```python
from build123d import *

# Parameters (mm, degrees)
ESBO_O1_R                = 87
RESSALTO_EXTRUS_O1_DEPTH = 2.5
CORTE_EXTRUS_O1_DEPTH    = 2.5
CORTE_EXTRUS_O2_START    = -2.5
ESBO_O3_W                = 27.5
ESBO_O3_H                = 33
CORTE_EXTRUS_O2_DEPTH    = 2.5
FILETE2_R                = 2
ESBO_O4_R                = 17
CORTE_EXTRUS_O3_DEPTH    = 4
CORTE_EXTRUS_O5_DEPTH    = 3
FURO_ROSCADO_DE_M2_51_D  = 2.05


with BuildPart() as part:
    # Esboço1 → Ressalto-extrusão1 (new body)
    with BuildSketch(Plane(origin=(0, 0, 0), x_dir=(1, 0, 0), z_dir=(0, 1, 0))):
        with Locations(Location((0, 0, 0), (0, 0, 270))):
            Circle(ESBO_O1_R)
    extrude(amount=RESSALTO_EXTRUS_O1_DEPTH)

    # Esboço2 → Corte-extrusão1 (cut)
    with BuildSketch(Plane(origin=(0, 2.5, 0), x_dir=(1, 0, 0), z_dir=(0, 1, 0))):
        Polygon((66.645866551, 55.922522043), (82.394162989, 37.154433186), (79.696950599, 34.891203265), (72.036506168, 28.463327168), (40.539913293, 65.999504881), (48.200357724, 72.427380978), (50.897570114, 74.690610899), align=None)
        Polygon((50.897570114, -74.690610899), (82.394162989, -37.154433186), (79.696950599, -34.891203265), (72.036506168, -28.463327168), (40.539913293, -65.999504881), (48.200357724, -72.427380978), align=None)
        Polygon((-72.036506168, 28.463327168), (-40.539913293, 65.999504881), (-48.200357724, 72.427380978), (-50.897570114, 74.690610899), (-66.645866551, 55.922522043), (-82.394162989, 37.154433186), (-79.696950599, 34.891203265), align=None)
        Polygon((-79.696950599, -34.891203265), (-82.394162989, -37.154433186), (-50.897570114, -74.690610899), (-48.200357724, -72.427380978), (-40.539913293, -65.999504881), (-72.036506168, -28.463327168), align=None)
    extrude(amount=-CORTE_EXTRUS_O1_DEPTH, mode=Mode.SUBTRACT)

    # Esboço3 → Corte-extrusão2 (cut)
    with BuildSketch(Plane(origin=(0, 2.5, 0), x_dir=(1, 0, 0), z_dir=(0, 1, 0)).offset(CORTE_EXTRUS_O2_START)):
        with Locations((-13.75, 58.5)):
            Rectangle(ESBO_O3_W, ESBO_O3_H)
        with Locations((13.75, 58.5)):
            Rectangle(ESBO_O3_W, ESBO_O3_H)
        with BuildLine():
            Line((0, 87), (0, 75))
            Line((0, 75), (27.5, 75))
            Line((27.5, 75), (44.09081537, 75))
            ThreePointArc((44.09081537, 75), (22.847319318, 83.946411478), (0, 87))
        make_face()
        with BuildLine():
            Line((-27.5, 75), (0, 75))
            Line((0, 75), (0, 87))
            ThreePointArc((0, 87), (-22.847319318, 83.946411478), (-44.09081537, 75))
            Line((-44.09081537, 75), (-27.5, 75))
        make_face()
    extrude(amount=CORTE_EXTRUS_O2_DEPTH, mode=Mode.SUBTRACT)

    # Filete2
    filete2_edges = [part.edges().sort_by_distance(p)[0] for p in [
        (27.5, 1.25, -42),
        (-27.5, 1.25, -42),
        (-27.5, 1.25, -75),
        (-44.09081537, 1.25, -75),
        (44.09081537, 1.25, -75),
        (27.5, 1.25, -75),
        (79.696950599, 1.25, 34.891203265),
        (72.036506168, 1.25, 28.463327168),
        (48.200357724, 1.25, 72.427380978),
        (40.539913293, 1.25, 65.999504881),
        (-79.696950599, 1.25, -34.891203265),
        (-72.036506168, 1.25, -28.463327168),
        (-48.200357724, 1.25, -72.427380978),
        (-40.539913293, 1.25, -65.999504881),
        (-79.696950599, 1.25, 34.891203265),
        (-48.200357724, 1.25, 72.427380978),
        (-40.539913293, 1.25, 65.999504881),
        (-72.036506168, 1.25, 28.463327168),
        (79.696950599, 1.25, -34.891203265),
        (48.200357724, 1.25, -72.427380978),
        (40.539913293, 1.25, -65.999504881),
        (72.036506168, 1.25, -28.463327168),
    ]]
    fillet(filete2_edges, radius=FILETE2_R)

    # Esboço4 → Corte-extrusão3 (cut)
    with BuildSketch(Plane(origin=(0, 2.5, 0), x_dir=(1, 0, 0), z_dir=(0, 1, 0))):
        with Locations(Location((61, 0, 0), (0, 0, 270))):
            Circle(ESBO_O4_R)
        with Locations(Location((-61, 0, 0), (0, 0, 270))):
            Circle(ESBO_O4_R)
    extrude(amount=-CORTE_EXTRUS_O3_DEPTH, mode=Mode.SUBTRACT)

    # Esboço7 → Corte-extrusão5 (cut)
    with BuildSketch(Plane(origin=(0, 2.5, 0), x_dir=(1, 0, 0), z_dir=(0, 1, 0))):
        with BuildLine():
            Line((-40.056146338, -19.904321081), (-26.557606535, -35.991254386))
            ThreePointArc((-26.557606535, -35.991254386), (-25.199829134, -36.698068563), (-23.739942429, -36.237768053))
            Line((-23.739942429, -36.237768053), (-7.653009124, -22.73922825))
            ThreePointArc((-7.653009124, -22.73922825), (-6.946194947, -21.381450849), (-7.406495457, -19.921564144))
            Line((-7.406495457, -19.921564144), (-20.90503526, -3.834630839))
            ThreePointArc((-20.90503526, -3.834630839), (-22.262812661, -3.127816662), (-23.722699366, -3.588117172))
            Line((-23.722699366, -3.588117172), (-39.809632672, -17.086656975))
            ThreePointArc((-39.809632672, -17.086656975), (-40.516446848, -18.444434376), (-40.056146338, -19.904321081))
        make_face()
        with BuildLine():
            Line((-23.722699366, 3.588117172), (-39.809632672, 17.086656975))
            ThreePointArc((-39.809632672, 17.086656975), (-40.516446848, 18.444434376), (-40.056146338, 19.904321081))
            Line((-40.056146338, 19.904321081), (-26.557606535, 35.991254386))
            ThreePointArc((-26.557606535, 35.991254386), (-25.199829134, 36.698068563), (-23.739942429, 36.237768053))
            Line((-23.739942429, 36.237768053), (-7.653009124, 22.73922825))
            ThreePointArc((-7.653009124, 22.73922825), (-6.946194947, 21.381450849), (-7.406495457, 19.921564144))
            Line((-7.406495457, 19.921564144), (-20.90503526, 3.834630839))
            ThreePointArc((-20.90503526, 3.834630839), (-22.262812661, 3.127816662), (-23.722699366, 3.588117172))
        make_face()
        with BuildLine():
            Line((40.056146338, 19.904321081), (26.557606535, 35.991254386))
            ThreePointArc((26.557606535, 35.991254386), (25.199829134, 36.698068563), (23.739942429, 36.237768053))
            Line((23.739942429, 36.237768053), (7.653009124, 22.73922825))
            ThreePointArc((7.653009124, 22.73922825), (6.946194947, 21.381450849), (7.406495457, 19.921564144))
            Line((7.406495457, 19.921564144), (20.90503526, 3.834630839))
            ThreePointArc((20.90503526, 3.834630839), (22.262812661, 3.127816662), (23.722699366, 3.588117172))
            Line((23.722699366, 3.588117172), (39.809632672, 17.086656975))
            ThreePointArc((39.809632672, 17.086656975), (40.516446848, 18.444434376), (40.056146338, 19.904321081))
        make_face()
        with BuildLine():
            Line((23.722699366, -3.588117172), (39.809632672, -17.086656975))
            ThreePointArc((39.809632672, -17.086656975), (40.516446848, -18.444434376), (40.056146338, -19.904321081))
            Line((40.056146338, -19.904321081), (26.557606535, -35.991254386))
            ThreePointArc((26.557606535, -35.991254386), (25.199829134, -36.698068563), (23.739942429, -36.237768053))
            Line((23.739942429, -36.237768053), (7.653009124, -22.73922825))
            ThreePointArc((7.653009124, -22.73922825), (6.946194947, -21.381450849), (7.406495457, -19.921564144))
            Line((7.406495457, -19.921564144), (20.90503526, -3.834630839))
            ThreePointArc((20.90503526, -3.834630839), (22.262812661, -3.127816662), (23.722699366, -3.588117172))
        make_face()
    extrude(amount=-CORTE_EXTRUS_O5_DEPTH, mode=Mode.SUBTRACT)

    # Furo roscado de M2.51 (through all)
    with Locations(Plane(origin=(-71, 2.5, -17.320508076), x_dir=(0, 0, 1), z_dir=(0, 1, 0))):
        with Locations((0, 0), (17.320508076, 30), (34.641016152, 0), (17.320508076, 112), (0, 142), (34.641016152, 142)):
            Hole(FURO_ROSCADO_DE_M2_51_D / 2)


solid = part.part
```
For this review, take the finished solid that the model builds, in its own axes (mm). A direction names the side the tool comes from. Round coordinates to 2 decimals unless told otherwise and drop trailing zeros. Loops run counter-clockwise (first coordinate to the right, second up) from the corner with the lowest first, then second, coordinate; pieces in that order, holes last.
Q1. Add section B-B on z = -13. Write out the cut boundary in (x, y).
Result sheet:
outline: (-86.02, 0) - (-71.95, 0) - (-71.95, 2.5) - (-86.02, 2.5) - close; (-50.05, 0) - (-34.94, 0) - (-34.94, 2.5) - (-50.05, 2.5) - close; (-13.21, 0) - (13.21, 0) - (13.21, 2.5) - (-13.21, 2.5) - close; (34.94, 0) - (50.05, 0) - (50.05, 2.5) - (34.94, 2.5) - close; (71.95, 0) - (86.02, 0) - (86.02, 2.5) - (71.95, 2.5) - close
Q2. Mouldability with a two-part tool opening along Z and no side actions: class faces 1 (the face through (-87, 1, 0)), 2 (the face through (46, 1, 8)), 3 (the face through (1, 2.5, 5)) as +Z half, -Z half, draft (parallel to the pull), parting line (faces both ways), or undercut.
Result sheet:
face 1: parting line
face 2: undercut
face 3: draft
Q3. Add section C-C on y = 1.4. Give the number of separate pieces and of enclosed holes in the cut face, plus the area to 3 significant figures.
Result sheet:
separate pieces: 1
enclosed holes: 12
area: 14,500 mm2
Q4. To check wall thickness, follow line 1 along X through (y, z) = (1.1, 12.5); line 2 along X through (y, z) = (2, 2.5); line 3 along Z through (x, y) = (-31.5, 0.15). State the ranges of each line that lie inside material, in increasing order.
Result sheet:
line 1: x = -86.1 to -72.52, -49.48 to -34.34, -13.63 to 13.63, 34.34 to 49.48, 72.52 to 86.1
line 2: x = -86.96 to -77.82, -44.18 to 44.18, 77.82 to 86.96
line 3: z = -75 to -30.1, -10.11 to 10.11, 30.1 to 81.1
Q5. Machinability: for faces 4 (the face through (87, 1, 0)), 5 (the face through (15.809, 1.268, 29.583)), which of the approach directions +Z, -Z, +X, -X, +Y, -Y give a long, thin tool a straight path to every point of the face, cutting with its end or side? Answer none if there is none.
Result sheet:
face 4: +X, +Y, -Y
face 5: +Y, -Y
Q6. Add section D-D on x = 58. Write out the cut boundary in (y, z), plus the area to 3 significant figures.
Result sheet:
outline: (0, -45.19) - (2.5, -45.19) - (2.5, -16.73) - (0, -16.73) - close; (0, 16.73) - (2.5, 16.73) - (2.5, 45.19) - (0, 45.19) - close
area: 142 mm2
Q7. Insertion check: pin 1 Ø0.8 at (y, z) = (1.5, -53) entering from +X; pin 2 Ø2.5 at (x, z) = (41, 0) entering from +Y; pin 3 Ø0.8 at (x, y) = (5, 1) entering from -Z; pin 4 Ø1 at (x, y) = (33.5, 1.5) entering from +Z. Each pin has a flat end and moves straight along its axis. Give the tip position at first contact, or say it passes through.
Result sheet:
pin 1: stops at x = 51.78
pin 2: stops at y = 2.5
pin 3: stops at z = -42
pin 4: stops at z = 80.5
Q8. Add section A-A on x = -61. Write out the cut boundary in (y, z).
Result sheet:
outline: (0, -41.62) - (2.5, -41.62) - (2.5, -17) - (0, -17) - close; (0, 17) - (2.5, 17) - (2.5, 41.62) - (0, 41.62) - close
